Design review of the part shown in the three views and the two pictorial views. Dimensions are in mm from the part's minimum x, y and z. A direction names the side the tool comes from. Round coordinates to 2 decimals unless told otherwise and drop trailing zeros. Write each loop counter-clockwise with the first axis right and the second up, starting at its lowest first coordinate (ties: lowest second). Pieces come first, ordered by that corner, then holes. Notation, with made-up numbers: (26.5, -14) -> (41.5, -14) arc R26 cw to (41.5, 24) -> close; hole circle Ø3 at (80, -20). An arc over 180 degrees is marked (long way). Return JSON: item names as keys, results as strings. Group by question number.
1. Take a section at B-B, the plane z = 8.5. Write out the cut boundary in (x, y).
2. For line 1 along X through (y, z) = (1, 18); line 2 along Z through (x, y) = (17, 2.5); line 3 along Y through (x, z) = (3, 28), list the stretches that pass through material, from the lowest coordinate up. Write a range as from..to.
3. Mouldability with a two-part tool opening along Z and no side actions: class the marked faces 1, 2 and 3 as pulls with the +Z half, pulls with the -Z half, needs draft (parallel to the pull), parting line crosses it, or undercut.
4. Take a section at D-D, the plane z = 4.5. Write out the cut boundary in (x, y).
5. Take a section at A-A, the plane x = 19. Write out the cut boundary in (y, z).
6. Clearance check with flat-ended pins moving along their axes: P1, Ø1.2, axis at x = 11, y = 14, coming from the -Z side; P2, Ø6, axis at x = 23, z = 31, coming from the -Y side; P3, Ø1.2, axis at y = 14, z = 22.5, coming from the +X side; P4, Ø1.9, axis at y = 14, z = 14, coming from the -X side. State where each tip first meets the part, or that it passes through.
7. Take a section at C-C, the plane y = 9.25. Write out the cut boundary in (x, z) (1 decimal), then the cut area to 3 significant figures.
8. Tool access review of the marked faces 4 and 5: name each direction out of +Z, -Z, +X, -X, +Y, -Y from which nothing blocks a thin tool from reaching the whole face with its end or side.
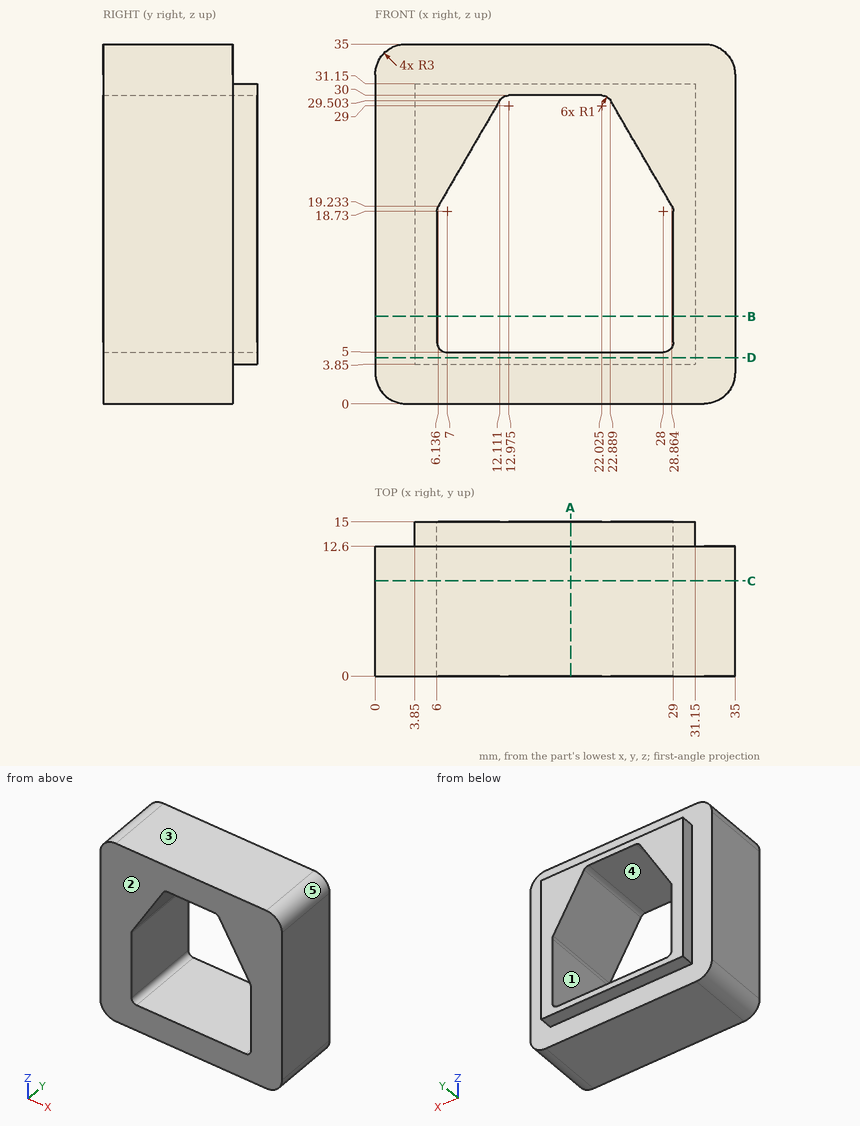
Output:
{
 "1": {"outline": "(0, 0) -> (6, 0) -> (6, 15) -> (3.85, 15) -> (3.85, 12.6) -> (0, 12.6) -> close; (29, 0) -> (35, 0) -> (35, 12.6) -> (31.15, 12.6) -> (31.15, 15) -> (29, 15) -> close"},
 "2": {"line 1": "x = 0..6, 29..35", "line 2": "z = 0..5, 30..35", "line 3": "y = 0..12.6"},
 "3": {"face 1": "undercut", "face 2": "needs draft", "face 3": "pulls with the +Z half"},
 "4": {"outline": "(0, 0) -> (35, 0) -> (35, 12.6) -> (31.15, 12.6) -> (31.15, 15) -> (3.85, 15) -> (3.85, 12.6) -> (0, 12.6) -> close"},
 "5": {"outline": "(0, 0) -> (12.6, 0) -> (12.6, 3.85) -> (15, 3.85) -> (15, 5) -> (0, 5) -> close; (0, 30) -> (15, 30) -> (15, 31.15) -> (12.6, 31.15) -> (12.6, 35) -> (0, 35) -> close"},
 "6": {"P1": "stops at z = 3.85", "P2": "stops at y = 0", "P3": "stops at x = 31.15", "P4": "stops at x = 3.85"},
 "7": {"outline": "(0, 3) arc R3 ccw to (3, 0) -> (32, 0) arc R3 ccw to (35, 3) -> (35, 32) arc R3 ccw to (32, 35) -> (3, 35) arc R3 ccw to (0, 32) -> close; hole (6, 6) arc R1 ccw to (7, 5) -> (28, 5) arc R1 ccw to (29, 6) -> (29, 18.7) arc R1 ccw to (28.9, 19.2) -> (22.9, 29.5) arc R1 ccw to (22, 30) -> (13, 30) arc R1 ccw to (12.1, 29.5) -> (6.1, 19.2) arc R1 ccw to (6, 18.7) -> close", "area": "713 mm^2"},
 "8": {"face 4": "+Y, -Y", "face 5": "+Z, +X, +Y, -Y"}
}
